Build history of the part. All positions in model axes, mm. Face numbers are marked on the shaded views. A direction names the side the tool comes from. Round coordinates to 2 decimals unless told otherwise and drop trailing zeros. Write each loop counter-clockwise with the first axis right and the second up, starting at its lowest first coordinate (ties: lowest second). Pieces come first, ordered by that corner, then holes.
from build123d import *

# Parameters (mm, degrees)
F1_DEPTH  = 12
F0_R      = 6.5
F0_R_2    = 3.25
F2_DEPTH  = 3
F4_START  = -4.35
F4_DEPTH  = 3.65
F5_D      = 3.3
F5_DEPTH  = 8
F5_TIP    = 0.9914200214
F6_D      = 6
F6_DEPTH  = 1.5
F6_TIP    = 1.8025818571
F8_START  = -4.35
F8_DEPTH  = 3.65
F9_D      = 6
F9_DEPTH  = 1.5
F9_TIP    = 1.8025818571
F10_D     = 3.3
F10_DEPTH = 8
F10_START = 2.3111618
F10_TIP   = 0.9914200214
F12_START = -4.35
F12_DEPTH = 3.65
F13_D     = 3.3
F13_DEPTH = 8
F13_TIP   = 0.9914200214
F14_D     = 6
F14_DEPTH = 1.5
F14_TIP   = 1.8025818571


with BuildPart() as f1:
    # F0 (on Front) → F1 (new body)
    with BuildSketch(Plane.XZ):
        with BuildLine():
            ThreePointArc((25.45, 11.749077978), (23.5832704407, 13.6158075373), (22.9, 16.1658075373))
            Line((22.9, 16.1658075373), (-22.9, 16.1658075373))
            ThreePointArc((-22.9, 16.1658075373), (-23.5832704407, 13.6158075373), (-25.45, 11.749077978))
            Line((-25.45, 11.749077978), (-2.55, -27.9148855153))
            ThreePointArc((-2.55, -27.9148855153), (0, -27.2316150746), (2.55, -27.9148855153))
            Line((2.55, -27.9148855153), (25.45, 11.749077978))
        make_face()
        with BuildLine():
            ThreePointArc((15.2679491924, 9.8149545762), (16.1339745962, 9.3149545762), (16.1339745962, 8.3149545762))
            Line((16.1339745962, 8.3149545762), (0.8660254038, -18.1299091524))
            ThreePointArc((0.8660254038, -18.1299091524), (0, -18.6299091524), (-0.8660254038, -18.1299091524))
            Line((-0.8660254038, -18.1299091524), (-16.1339745962, 8.3149545762))
            ThreePointArc((-16.1339745962, 8.3149545762), (-16.1339745962, 9.3149545762), (-15.2679491924, 9.8149545762))
            Line((-15.2679491924, 9.8149545762), (15.2679491924, 9.8149545762))
        make_face(mode=Mode.SUBTRACT)
    extrude(amount=F1_DEPTH)



with BuildPart() as f1b:
    # F0 (on Front) → F1, piece 2 (new body)
    with BuildSketch(Plane.XZ):
        Circle(F0_R)
        Circle(F0_R_2, mode=Mode.SUBTRACT)
    extrude(amount=F1_DEPTH)


with BuildPart() as f1_1:
    add(f1.part)

    add(f1b.part)  # F2 merges F1b
    # F0 (on Front) → F2 (join)
    with BuildSketch(Plane.XZ):
        with BuildLine():
            Line((0.8660254038, -18.1299091524), (16.1339745962, 8.3149545762))
            ThreePointArc((16.1339745962, 8.3149545762), (16.1339745962, 9.3149545762), (15.2679491924, 9.8149545762))
            Line((15.2679491924, 9.8149545762), (-15.2679491924, 9.8149545762))
            ThreePointArc((-15.2679491924, 9.8149545762), (-16.1339745962, 9.3149545762), (-16.1339745962, 8.3149545762))
            Line((-16.1339745962, 8.3149545762), (-0.8660254038, -18.1299091524))
            ThreePointArc((-0.8660254038, -18.1299091524), (0, -18.6299091524), (0.8660254038, -18.1299091524))
        make_face()
        Circle(F0_R, mode=Mode.SUBTRACT)
    extrude(amount=F2_DEPTH)

    # F3 (on face) → F4 (cut)
    with BuildSketch(Plane.XY.offset(16.1658075373).offset(F4_START)):
        Polygon((-6.8256842194, -8.9), (-5.1513684387, -6), (-6.8256842194, -3.1), (-10.1743157806, -3.1), (-11.8486315613, -6), (-10.1743157806, -8.9), align=None)
        Polygon((10.1743157806, -8.9), (11.8486315613, -6), (10.1743157806, -3.1), (6.8256842194, -3.1), (5.1513684387, -6), (6.8256842194, -8.9), align=None)
    extrude(amount=-F4_DEPTH, mode=Mode.SUBTRACT)

    # F5
    with Locations(Plane.XY.offset(16.1658075373)):
        with Locations((8.5, -6), (-8.5, -6)):
            Hole(F5_D / 2, depth=F5_DEPTH)
            with Locations((0, 0, -(F5_DEPTH + F5_TIP / 2))):  # 118° drill point
                Cone(0, F5_D / 2, F5_TIP, mode=Mode.SUBTRACT)

    # F6
    with Locations(Plane.XY.offset(16.1658075373)):
        with Locations((8.5, -6), (-8.5, -6)):
            Hole(F6_D / 2, depth=F6_DEPTH)
            with Locations((0, 0, -(F6_DEPTH + F6_TIP / 2))):  # 118° drill point
                Cone(0, F6_D / 2, F6_TIP, mode=Mode.SUBTRACT)

    # F7 (on face) → F8 (cut)
    with BuildSketch(Plane(origin=(-14, 0, -8.0829037687), x_dir=(0, -1, 0), z_dir=(-0.8660254038, 0, -0.5)).offset(F8_START)):
        Polygon((3.1, 6.8256842194), (6, 5.1513684387), (8.9, 6.8256842194), (8.9, 10.1743157806), (6, 11.8486315613), (3.1, 10.1743157806), align=None)
        Polygon((3.1, -10.1743157806), (6, -11.8486315613), (8.9, -10.1743157806), (8.9, -6.8256842194), (6, -5.1513684387), (3.1, -6.8256842194), align=None)
    extrude(amount=-F8_DEPTH, mode=Mode.SUBTRACT)

    # F9
    with Locations(Plane(origin=(-14, 0, -8.0829037687), x_dir=(0, -1, 0), z_dir=(-0.8660254038, 0, -0.5))):
        with Locations((6, 8.5), (6, -8.5)):
            Hole(F9_D / 2, depth=F9_DEPTH)
            with Locations((0, 0, -(F9_DEPTH + F9_TIP / 2))):  # 118° drill point
                Cone(0, F9_D / 2, F9_TIP, mode=Mode.SUBTRACT)

    # F10
    # its depths count from where the whole tool has entered the part; down to there all is cleared
    with Locations(Plane(origin=(-14, 0, -8.0829037687), x_dir=(0, -1, 0), z_dir=(-0.8660254038, 0, -0.5)).offset(-F10_START)):
        with Locations((6, 8.5), (6, -8.5)):
            Hole(F10_D / 2, depth=F10_DEPTH)
            with Locations((0, 0, -(F10_DEPTH + F10_TIP / 2))):  # 118° drill point
                Cone(0, F10_D / 2, F10_TIP, mode=Mode.SUBTRACT)

    # F11 (on face) → F12 (cut)
    with BuildSketch(Plane(origin=(14, 0, -8.0829037687), x_dir=(0, 1, 0), z_dir=(0.8660254038, 0, -0.5)).offset(F12_START)):
        Polygon((-3.1, -6.8256842194), (-6, -5.1513684387), (-8.9, -6.8256842194), (-8.9, -10.1743157806), (-6, -11.8486315613), (-3.1, -10.1743157806), align=None)
        Polygon((-3.1, 6.8256842194), (-3.1, 10.1743157806), (-6, 11.8486315613), (-8.9, 10.1743157806), (-8.9, 6.8256842194), (-6, 5.1513684387), align=None)
    extrude(amount=-F12_DEPTH, mode=Mode.SUBTRACT)

    # F13
    with Locations(Plane(origin=(14, 0, -8.0829037687), x_dir=(0, 1, 0), z_dir=(0.8660254038, 0, -0.5))):
        with Locations((-6, -8.5), (-6, 8.5)):
            Hole(F13_D / 2, depth=F13_DEPTH)
            with Locations((0, 0, -(F13_DEPTH + F13_TIP / 2))):  # 118° drill point
                Cone(0, F13_D / 2, F13_TIP, mode=Mode.SUBTRACT)

    # F14
    with Locations(Plane(origin=(14, 0, -8.0829037687), x_dir=(0, 1, 0), z_dir=(0.8660254038, 0, -0.5))):
        with Locations((-6, -8.5), (-6, 8.5)):
            Hole(F14_D / 2, depth=F14_DEPTH)
            with Locations((0, 0, -(F14_DEPTH + F14_TIP / 2))):  # 118° drill point
                Cone(0, F14_D / 2, F14_TIP, mode=Mode.SUBTRACT)


solid = f1_1.part
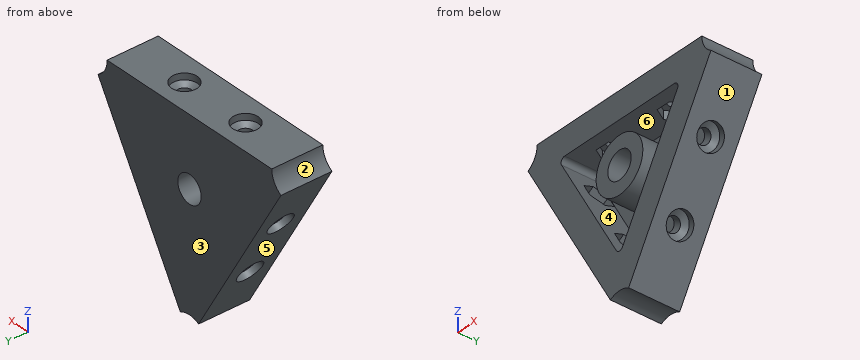
1) Slice it at C-C (y = -2). Write the cut outline in (x, z).
Results:
outline: (-25.45, 11.75) - (-2.55, -27.91) arc R5.1 cw to (2.55, -27.91) - (25.45, 11.75) arc R5.1 cw to (22.9, 16.17) - (-22.9, 16.17) arc R5.1 cw to start; hole circle Ø6.5 at (0, 0)
2) Slice it at A-A (x = 0). Write the cut outline in (y, z), plus the area to 3 significant figures.
Results:
outline: (-12, -27.23) - (0, -27.23) - (0, -3.25) - (-12, -3.25) - (-12, -6.5) - (-3, -6.5) - (-3, -18.63) - (-12, -18.63) - close; (-12, 3.25) - (0, 3.25) - (0, 16.17) - (-12, 16.17) - (-12, 9.81) - (-3, 9.81) - (-3, 6.5) - (-12, 6.5) - close
area: 304 mm2
3) Wall check: L1, parallel to Z at x = 0, y = -7.25; L2, parallel to Z at x = -7, y = -7.75; L3, parallel to Y at x = 8.5, z = 13.05. Give the ranges that are in metal, low to high.
Results:
L1: z = -27.23 to -18.63, -6.5 to -3.25, 3.25 to 6.5, 9.81 to 16.17
L2: z = -20.21 to -11.51, -11.16 to -7.51, 11.82 to 14.25
L3: y = -12 to -7.65, -4.35 to 0
4) Slice it at B-B (y = -9.75). Write the cut outline in (x, z).
Results:
outline: (-25.45, 11.75) - (-2.55, -27.91) arc R5.1 cw to (2.55, -27.91) - (25.45, 11.75) arc R5.1 cw to (22.9, 16.17) - (-22.9, 16.17) arc R5.1 cw to start; circle Ø13 at (0, 0); hole (-16.13, 8.31) - (-0.87, -18.13) arc R1 ccw to (0.87, -18.13) - (16.13, 8.31) arc R1 ccw to (15.27, 9.81) - (-15.27, 9.81) arc R1 ccw to start; hole circle Ø6.5 at (0, 0)
5) Slice it at D-D (z = -19.5). Write the cut outline in (x, y).
Results:
outline: (-7.41, -12) - (7.41, -12) - (7.41, 0) - (-7.41, 0) - close
6) Which spindle directions (+Z, -Z, +X, -X, +Y, -Y) get a long thin tool onto all of the face, cutting with end or side? Do the marked faces 5 and 6. Say none if no direction does.
Results:
face 5: -Z, -X, +Y, -Y
face 6: -Y
7) Pin check, flat tips, straight feed: pin 1 Ø7 at (x, y) = (5, -6) entering from -Z; pin 2 Ø7 at (x, y) = (8.5, -6) entering from -Z; pin 3 Ø1 at (y, z) = (-5, -17.5) entering from +X. Stop position of each tip, or through.
Results:
pin 1: stops at z = -27.91
pin 2: stops at z = -23.67
pin 3: stops at x = 8.44
8) Mould opens along Z. For the marked faces 1, 2, 3 and 4 say: released by +Z, released by -Z, zero draft, split by the parting line, or undercut.
Results:
face 1: released by -Z
face 2: released by +Z
face 3: zero draft
face 4: undercut
